CAD build for the part. Positions are in the model's coordinates, mm. Face numbers are marked on the shaded views. Round coordinates to 2 decimals unless told otherwise and drop trailing zeros. Loops run counter-clockwise (first coordinate to the right, second up) from the corner with the lowest first, then second, coordinate; pieces in that order, holes last. Notation, with made-up numbers: (-38.75, -40) -> (15.25, -40) arc R10 ccw to (15.25, -29) -> close; hole circle Ø4 at (60.25, 1). An arc over 180 degrees is marked (long way). Answer as CSV lines item,"result".
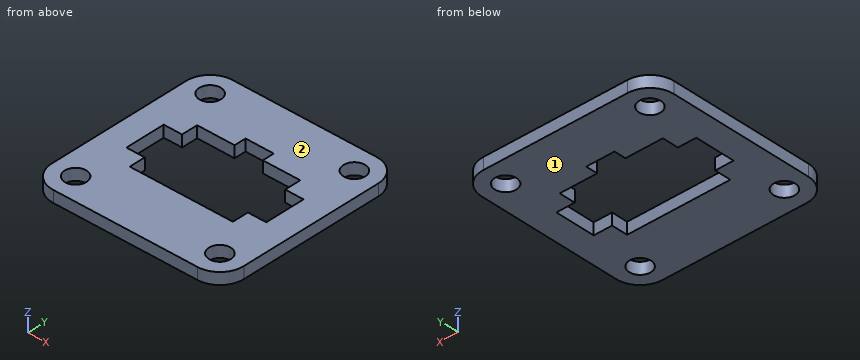
```python
from build123d import *

# Parameters (mm, degrees)
SKETCH1_W           = 26
SKETCH1_H           = 26
BOSS_EXTRUDE1_DEPTH = 1.5875
CUT_EXTRUDE1_DEPTH  = 37.803806274
FILLET1_R           = 3.175
SKETCH5_R           = 1.55
CUT_EXTRUDE2_DEPTH  = 37.803806274
MOVE_FACE1_BY       = 0.0762
MOVE_FACE1_2_BY     = 0.0762
MOVE_FACE1_3_BY     = 0.0762
MOVE_FACE1_4_BY     = 0.0762
MOVE_FACE1_5_BY     = 0.0762
MOVE_FACE1_6_BY     = 0.0762
MOVE_FACE1_7_BY     = 0.0762
MOVE_FACE1_8_BY     = 0.0762
MOVE_FACE1_9_BY     = 0.0762
MOVE_FACE1_10_BY    = 0.0762
MOVE_FACE1_11_BY    = 0.0762
MOVE_FACE1_12_BY    = 0.0762
MOVE_FACE1_13_BY    = 0.0762
MOVE_FACE1_14_BY    = 0.0762
MOVE_FACE1_15_BY    = 0.0762
MOVE_FACE1_16_BY    = 0.0762
MOVE_FACE1_17_BY    = 0.0762
MOVE_FACE1_18_BY    = 0.0762
MOVE_FACE1_19_BY    = 0.0762
MOVE_FACE1_20_BY    = 0.0762
MOVE_FACE1_21_BY    = 0.0762
MOVE_FACE1_22_BY    = 0.0762
MOVE_FACE1_23_BY    = 0.0762
MOVE_FACE1_24_BY    = 0.0762
MOVE_FACE1_25_BY    = 0.0762
MOVE_FACE1_26_BY    = 0.0762
MOVE_FACE1_27_BY    = 0.0762
MOVE_FACE1_28_BY    = 0.0762


with BuildPart() as part:
    # Sketch1 → Boss-Extrude1 (new body)
    with BuildSketch(Plane.XY):
        with Locations((13, 13)):
            Rectangle(SKETCH1_W, SKETCH1_H)
    extrude(amount=BOSS_EXTRUDE1_DEPTH)

    # Sketch2 → Cut-Extrude1 (cut, through all)
    with BuildSketch(Plane.XY.offset(1.5875)):
        Polygon((5.9, 8), (5.9, 10.2), (3.4, 10.2), (3.4, 15.8), (5.9, 15.8), (5.9, 18), (11, 18), (11, 19.6), (15, 19.6), (15, 18), (20.1, 18), (20.1, 15.8), (22.6, 15.8), (22.6, 10.2), (20.1, 10.2), (20.1, 8), align=None)
    extrude(amount=-CUT_EXTRUDE1_DEPTH, mode=Mode.SUBTRACT)

    # Fillet1
    fillet1_edges = [part.edges().sort_by_distance(p)[0] for p in [
        (0, 26, 0.79375),
        (26, 26, 0.79375),
        (26, 0, 0.79375),
        (0, 0, 0.79375),
    ]]
    fillet(fillet1_edges, radius=FILLET1_R)

    # Sketch5 → Cut-Extrude2 (cut, through all)
    with BuildSketch(Plane.XY.offset(1.5875)):
        with Locations((3.175, 22.825)):
            Circle(SKETCH5_R)
        with Locations((22.825, 22.825)):
            Circle(SKETCH5_R)
        with Locations((22.825, 3.175)):
            Circle(SKETCH5_R)
        with Locations((3.175, 3.175)):
            Circle(SKETCH5_R)
    extrude(amount=-CUT_EXTRUDE2_DEPTH, mode=Mode.SUBTRACT)

    # Move Face1: a curved face moved outward by 0.0762
    add(Solid.thicken(part.faces().sort_by_distance((25.07006403, 0.92993597, 0.79375))[0], MOVE_FACE1_BY))

    # Move Face1 2: a face moved outward by 0.0762
    extrude(part.faces().sort_by_distance((26, 13, 0.79375))[0], amount=MOVE_FACE1_2_BY, dir=(1, 0, 0))

    # Move Face1 3: a face moved outward by 0.0762
    extrude(part.faces().sort_by_distance((13, 26, 0.79375))[0], amount=MOVE_FACE1_3_BY, dir=(0, 1, 0))

    # Move Face1 4: a curved face moved outward by 0.0762
    add(Solid.thicken(part.faces().sort_by_distance((25.07006403, 25.07006403, 0.79375))[0], MOVE_FACE1_4_BY))

    # Move Face1 5: a curved face moved outward by 0.0762
    add(Solid.thicken(part.faces().sort_by_distance((0.92993597, 25.07006403, 0.79375))[0], MOVE_FACE1_5_BY))

    # Move Face1 6: a face moved outward by 0.0762
    extrude(part.faces().sort_by_distance((0, 13, 0.79375))[0], amount=MOVE_FACE1_6_BY, dir=(-1, 0, 0))

    # Move Face1 7: a face moved outward by 0.0762
    extrude(part.faces().sort_by_distance((13, 0, 0.79375))[0], amount=MOVE_FACE1_7_BY, dir=(0, -1, 0))

    # Move Face1 8: a curved face moved outward by 0.0762
    add(Solid.thicken(part.faces().sort_by_distance((0.92993597, 0.92993597, 0.79375))[0], MOVE_FACE1_8_BY))

    # Move Face1 9: a curved face moved outward by 0.0762
    add(Solid.thicken(part.faces().sort_by_distance((1.625, 3.175, 0.79375))[0], MOVE_FACE1_9_BY))

    # Move Face1 10: a curved face moved outward by 0.0762
    add(Solid.thicken(part.faces().sort_by_distance((1.625, 22.825, 0.79375))[0], MOVE_FACE1_10_BY))

    # Move Face1 11: a curved face moved outward by 0.0762
    add(Solid.thicken(part.faces().sort_by_distance((21.275, 22.825, 0.79375))[0], MOVE_FACE1_11_BY))

    # Move Face1 12: a curved face moved outward by 0.0762
    add(Solid.thicken(part.faces().sort_by_distance((21.275, 3.175, 0.79375))[0], MOVE_FACE1_12_BY))

    # Move Face1 13: a face moved outward by 0.0762
    extrude(part.faces().sort_by_distance((21.35, 10.2, 0.79375))[0], amount=MOVE_FACE1_13_BY, dir=(0, 1, 0))

    # Move Face1 14: a face moved outward by 0.0762
    extrude(part.faces().sort_by_distance((4.65, 10.2, 0.79375))[0], amount=MOVE_FACE1_14_BY, dir=(0, 1, 0))

    # Move Face1 15: a face moved outward by 0.0762
    extrude(part.faces().sort_by_distance((5.9, 9.1, 0.79375))[0], amount=MOVE_FACE1_15_BY, dir=(1, 0, 0))

    # Move Face1 16: a face moved outward by 0.0762
    extrude(part.faces().sort_by_distance((3.4, 13, 0.79375))[0], amount=MOVE_FACE1_16_BY, dir=(1, 0, 0))

    # Move Face1 17: a face moved outward by 0.0762
    extrude(part.faces().sort_by_distance((5.9, 16.9, 0.79375))[0], amount=MOVE_FACE1_17_BY, dir=(1, 0, 0))

    # Move Face1 18: a face moved outward by 0.0762
    extrude(part.faces().sort_by_distance((11, 18.8, 0.79375))[0], amount=MOVE_FACE1_18_BY, dir=(1, 0, 0))

    # Move Face1 19: a face moved outward by 0.0762
    extrude(part.faces().sort_by_distance((13, 8, 0.79375))[0], amount=MOVE_FACE1_19_BY, dir=(0, 1, 0))

    # Move Face1 20: a face moved outward by 0.0762
    extrude(part.faces().sort_by_distance((20.1, 9.1, 0.79375))[0], amount=MOVE_FACE1_20_BY, dir=(-1, 0, 0))

    # Move Face1 21: a face moved outward by 0.0762
    extrude(part.faces().sort_by_distance((22.6, 13, 0.79375))[0], amount=MOVE_FACE1_21_BY, dir=(-1, 0, 0))

    # Move Face1 22: a face moved outward by 0.0762
    extrude(part.faces().sort_by_distance((20.1, 16.9, 0.79375))[0], amount=MOVE_FACE1_22_BY, dir=(-1, 0, 0))

    # Move Face1 23: a face moved outward by 0.0762
    extrude(part.faces().sort_by_distance((15, 18.8, 0.79375))[0], amount=MOVE_FACE1_23_BY, dir=(-1, 0, 0))

    # Move Face1 24: a face moved outward by 0.0762
    extrude(part.faces().sort_by_distance((13, 19.6, 0.79375))[0], amount=MOVE_FACE1_24_BY, dir=(0, -1, 0))

    # Move Face1 25: a face moved outward by 0.0762
    extrude(part.faces().sort_by_distance((4.65, 15.8, 0.79375))[0], amount=MOVE_FACE1_25_BY, dir=(0, -1, 0))

    # Move Face1 26: a face moved outward by 0.0762
    extrude(part.faces().sort_by_distance((8.45, 18, 0.79375))[0], amount=MOVE_FACE1_26_BY, dir=(0, -1, 0))

    # Move Face1 27: a face moved outward by 0.0762
    extrude(part.faces().sort_by_distance((17.55, 18, 0.79375))[0], amount=MOVE_FACE1_27_BY, dir=(0, -1, 0))

    # Move Face1 28: a face moved outward by 0.0762
    extrude(part.faces().sort_by_distance((21.35, 15.8, 0.79375))[0], amount=MOVE_FACE1_28_BY, dir=(0, -1, 0))


solid = part.part
```
Q1. Slice it at D-D, the plane x = 23.25. Give the cut face in (y, z).
Results:
outline,"(-0.05, 0) -> (1.76, 0) -> (1.76, 1.59) -> (-0.05, 1.59) -> close; (4.59, 0) -> (21.41, 0) -> (21.41, 1.59) -> (4.59, 1.59) -> close; (24.24, 0) -> (26.05, 0) -> (26.05, 1.59) -> (24.24, 1.59) -> close"
Q2. Slice it at B-B, the plane x = 19. Give the cut face in (y, z).
Results:
outline,"(-0.08, 0) -> (8.08, 0) -> (8.08, 1.59) -> (-0.08, 1.59) -> close; (17.92, 0) -> (26.08, 0) -> (26.08, 1.59) -> (17.92, 1.59) -> close"
Q3. Two-plate mould, pull along Z, no slides. Class the marked faces 1 and 2: pulls with the +Z half, pulls with the -Z half, needs draft (parallel to the pull), parting line crosses it, or undercut.
Results:
face 1,"pulls with the -Z half"
face 2,"pulls with the +Z half"
Q4. Slice it at A-A, the plane y = 11.5. Give the cut face in (x, z), and give its area (3 significant figures).
Results:
outline,"(-0.08, 0) -> (3.48, 0) -> (3.48, 1.59) -> (-0.08, 1.59) -> close; (22.52, 0) -> (26.08, 0) -> (26.08, 1.59) -> (22.52, 1.59) -> close"
area,"11.3 mm2"
Q5. Slice it at C-C, the plane z = 0.5. Give the cut face in (x, y) (3 decimals).
Results:
outline,"(-0.076, 3.175) arc R3.251 ccw to (3.175, -0.076) -> (22.825, -0.076) arc R3.251 ccw to (26.076, 3.175) -> (26.076, 22.825) arc R3.251 ccw to (22.825, 26.076) -> (3.175, 26.076) arc R3.251 ccw to (-0.076, 22.825) -> close; hole circle Ø2.948 at (3.175, 3.175); hole circle Ø2.948 at (3.175, 22.825); hole (3.476, 10.276) -> (5.976, 10.276) -> (5.976, 8.076) -> (20.024, 8.076) -> (20.024, 10.276) -> (22.524, 10.276) -> (22.524, 15.724) -> (20.024, 15.724) -> (20.024, 17.924) -> (14.924, 17.924) -> (14.924, 19.524) -> (11.076, 19.524) -> (11.076, 17.924) -> (5.976, 17.924) -> (5.976, 15.724) -> (3.476, 15.724) -> close; hole circle Ø2.948 at (22.825, 3.175); hole circle Ø2.948 at (22.825, 22.825)"
Q6. Probe L1, parallel to X at y = 14.75, z = 0.2; L2, parallel to X at y = 9.75, z = 1.15; L3, parallel to Y at x = 20.5, z = 0.9. List the from-to ranges inside material, lowest first. Write a range as [from, to].
Results:
L1,"[-0.08, 3.48], [22.52, 26.08]"
L2,"[-0.08, 5.98], [20.02, 26.08]"
L3,"[-0.08, 10.28], [15.72, 26.08]"
Q7. Drop a flat-ended pin along its axis: pin 1 Ø2.5 at (x, y) = (22.825, 3.175) entering from -Z (3 decimals). Give the stop position or say it passes through.
Results:
pin 1,"through"
